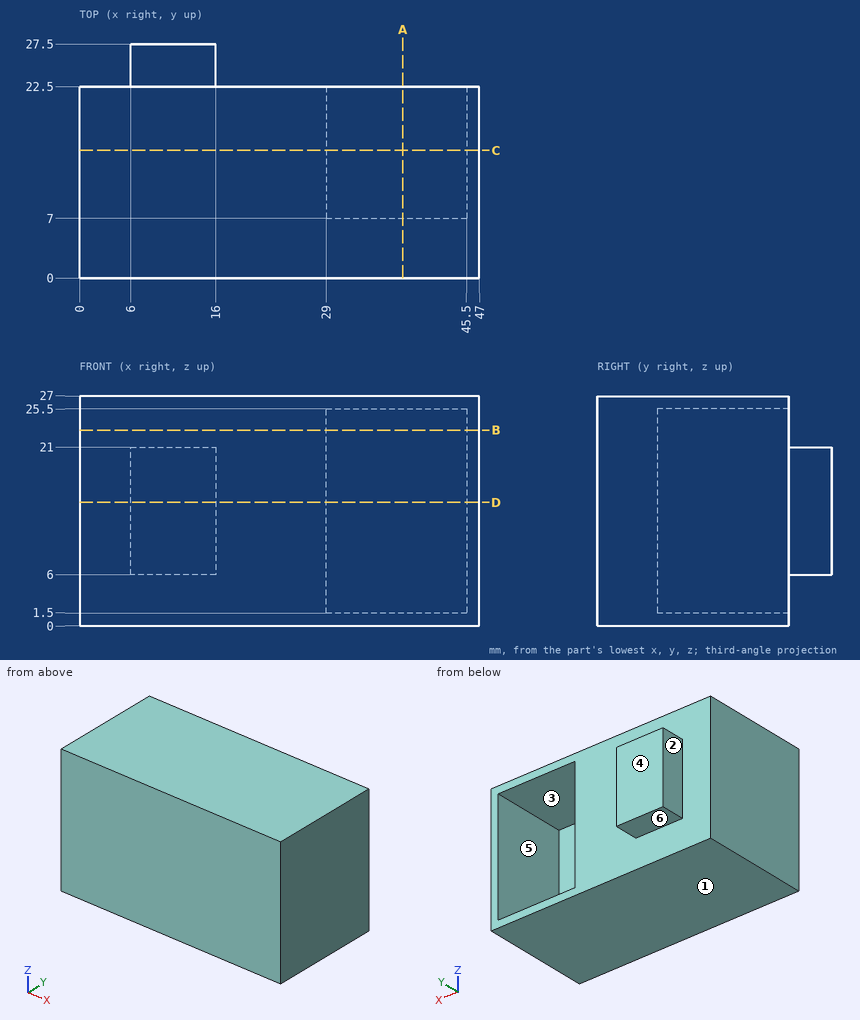
Geometry: see drawing. Coordinates: mm, zero at the bounding-box minimum. A direction names the side the tool comes from. Round coordinates to 2 decimals unless told otherwise and drop trailing zeros. Write each loop counter-clockwise with the first axis right and the second up, starting at its lowest first coordinate (ties: lowest second). Pieces come first, ordered by that corner, then holes. Notation, with made-up numbers: (-39, 88.5) -> (-4, 88.5) arc R17 ccw to (-4, 110.5) -> close; hole circle Ø4 at (84.5, 22). An arc over 180 degrees is marked (long way). Answer as CSV lines item,"result".
1. Section A-A (x = 38). Return the cut outline in (y, z).
Geometry says:
outline,"(0, 0) -> (22.5, 0) -> (22.5, 1.5) -> (7, 1.5) -> (7, 25.5) -> (22.5, 25.5) -> (22.5, 27) -> (0, 27) -> close"
2. Section D-D (z = 14.5). Return the cut outline in (x, y).
Geometry says:
outline,"(0, 0) -> (47, 0) -> (47, 22.5) -> (45.5, 22.5) -> (45.5, 7) -> (29, 7) -> (29, 22.5) -> (16, 22.5) -> (16, 27.5) -> (6, 27.5) -> (6, 22.5) -> (0, 22.5) -> close"
3. Section B-B (z = 23). Return the cut outline in (x, y).
Geometry says:
outline,"(0, 0) -> (47, 0) -> (47, 22.5) -> (45.5, 22.5) -> (45.5, 7) -> (29, 7) -> (29, 22.5) -> (0, 22.5) -> close"
4. Section C-C (y = 15). Return the cut outline in (x, z), plus the area to 3 significant figures.
Geometry says:
outline,"(0, 0) -> (47, 0) -> (47, 27) -> (0, 27) -> close; hole (29, 1.5) -> (45.5, 1.5) -> (45.5, 25.5) -> (29, 25.5) -> close"
area,"873 mm^2"
5. Contact query for flat-ended pins moving along their axis: P1, Ø4, axis at x = 9, y = 26, coming from the +Z side; P2, Ø5, axis at x = 41.5, z = 9.5, coming from the +Y side; P3, Ø3, axis at x = 26.5, z = 17, coming from the +Y side. Output: stop coordinate, or through.
Geometry says:
P1,"stops at z = 21"
P2,"stops at y = 7"
P3,"stops at y = 22.5"
6. Ray query, L1, parallel to X at y = 20.75, z = 4.75; L2, parallel to Z at x = 45, y = 12.75; L3, parallel to Y at x = 3, z = 12. Return the intervals inside material, ascending. Write a range as [from, to].
Geometry says:
L1,"x = [0, 29], [45.5, 47]"
L2,"z = [0, 1.5], [25.5, 27]"
L3,"y = [0, 22.5]"
7. Mould query, pull axis Z, two halves, no side actions, for the marked faces 4, 5 and 6. Classes: +Z half, -Z half, draft (parallel to the pull), parting line (faces both ways), or undercut.
Geometry says:
face 4,"draft"
face 5,"undercut"
face 6,"-Z half"
8. Reachability of the marked faces 1, 2 and 3 from +Z, -Z, +X, -X, +Y, -Y: full face, straight path, thin tool, end or side. Return the list, or none.
Geometry says:
face 1,"-Z, +X, -X, +Y, -Y"
face 2,"+Z, -Z, -X, +Y"
face 3,"+Y"
